```python
from build123d import *

# Parameters (mm, degrees)
SKETCH1_W                = 220
SKETCH1_H                = 170
BOSS_EXTRUDE1_DEPTH      = 100
SKETCH3_W                = 200
SKETCH3_H                = 150
CUT_EXTRUDE2_DEPTH       = 90
FILLET1_R                = 10
SKETCH4_W                = 130
SKETCH4_H                = 90
CUT_EXTRUDE3_DEPTH       = 10
SKETCH8_W                = 223.528125383
SKETCH8_H                = 171.877504909
CUT_EXTRUDE5_DEPTH       = 10
CUT_EXTRUDE7_REACH       = 505.38
SKETCH9_R                = 7.5
CUT_EXTRUDE8_REACH       = 505.38
SKETCH10_W               = 50
SKETCH10_H               = 30
CUT_EXTRUDE9_REACH       = 384.733
SKETCH11_W               = 20
SKETCH11_H               = 1
CUT_EXTRUDE10_REACH      = 505.38
CUT_EXTRUDE11_DEPTH      = 10
CUT_EXTRUDE12_REACH      = 505.38
SKETCH15_R               = 5.863278905
CUT_EXTRUDE13_DEPTH      = 8
BOSS_EXTRUDE3_DEPTH      = 8
BOSS_EXTRUDE3_DEPTH_BACK = 3
SKETCH16_R               = 1.3
SKETCH17_R               = 13.825952239
SKETCH17_R_2             = 5.825952239
EXTRUDE_THIN1_DEPTH      = 8
FILLET2_R                = 8
SKETCH18_W               = 15
SKETCH18_H               = 21
CUT_EXTRUDE14_DEPTH      = 249


with BuildPart() as part:
    # Sketch1 → Boss-Extrude1 (new body)
    with BuildSketch(Plane.XY):
        with Locations((-355.179344655, 214.973620006)):
            Rectangle(SKETCH1_W, SKETCH1_H)
    extrude(amount=BOSS_EXTRUDE1_DEPTH)

    # Sketch3 → Cut-Extrude2 (cut)
    with BuildSketch(Plane.XY.offset(100)):
        with Locations((-355.179344655, 214.973620006)):
            Rectangle(SKETCH3_W, SKETCH3_H)
    extrude(amount=-CUT_EXTRUDE2_DEPTH, mode=Mode.SUBTRACT)

    # Fillet1
    fillet1_edges = [part.edges().sort_by_distance(p)[0] for p in [
        (-355.179344655, 299.973620006, 0),
        (-245.179344655, 214.973620006, 0),
        (-355.179344655, 129.973620006, 0),
        (-465.179344655, 214.973620006, 0),
    ]]
    fillet(fillet1_edges, radius=FILLET1_R)

    # Sketch4 → Cut-Extrude3 (cut)
    with BuildSketch(Plane(origin=(0, 299.973620006, 0), x_dir=(1, 0, 0), z_dir=(0, 1, 0))):
        with Locations((-330.179344655, -55)):
            Rectangle(SKETCH4_W, SKETCH4_H)
    extrude(amount=-CUT_EXTRUDE3_DEPTH, mode=Mode.SUBTRACT)

    # Sketch8 → Cut-Extrude5 (cut)
    with BuildSketch(Plane.XY.offset(90)):
        with Locations((-354.80209528, 215.143634814)):
            Rectangle(SKETCH8_W, SKETCH8_H)
    extrude(amount=CUT_EXTRUDE5_DEPTH, mode=Mode.SUBTRACT)

    # Sketch9 → Cut-Extrude7 (cut, up to next)
    with BuildSketch(Plane.XZ.offset(-129.973620006), mode=Mode.PRIVATE) as cut_extrude7_sk1:
        with Locations(Location((-445.179344655, 30, 0), (0, 0, 270))):
            Circle(SKETCH9_R)
    cut_extrude7_tool1 = extrude(cut_extrude7_sk1.sketch, amount=-CUT_EXTRUDE7_REACH, mode=Mode.PRIVATE) & part.part
    add(cut_extrude7_tool1.solids().sort_by_distance((-445.179345, 129.97362, 30))[0], mode=Mode.SUBTRACT)

    # Sketch10 → Cut-Extrude8 (cut, up to next)
    with BuildSketch(Plane.XZ.offset(-129.973620006), mode=Mode.PRIVATE) as cut_extrude8_sk1:
        with Locations((-282.179344655, 35)):
            Rectangle(SKETCH10_W, SKETCH10_H)
    cut_extrude8_tool1 = extrude(cut_extrude8_sk1.sketch, amount=-CUT_EXTRUDE8_REACH, mode=Mode.PRIVATE) & part.part
    add(cut_extrude8_tool1.solids().sort_by_distance((-282.179345, 129.97362, 35))[0], mode=Mode.SUBTRACT)

    # Sketch11 → Cut-Extrude9 (cut, up to next)
    with BuildSketch(Plane.ZY.offset(465.179344655), mode=Mode.PRIVATE) as cut_extrude9_sk1:
        with Locations((30.04058668, 161.535899553)):
            Rectangle(SKETCH11_W, SKETCH11_H)
    cut_extrude9_tool1 = extrude(cut_extrude9_sk1.sketch, amount=-CUT_EXTRUDE9_REACH, mode=Mode.PRIVATE) & part.part
    # Sketch11 → Cut-Extrude9 (cut, up to next)
    with BuildSketch(Plane.ZY.offset(465.179344655), mode=Mode.PRIVATE) as cut_extrude9_sk2:
        with Locations((30.04058668, 156.535899553)):
            Rectangle(SKETCH11_W, SKETCH11_H)
    cut_extrude9_tool2 = extrude(cut_extrude9_sk2.sketch, amount=-CUT_EXTRUDE9_REACH, mode=Mode.PRIVATE) & part.part
    # Sketch11 → Cut-Extrude9 (cut, up to next)
    with BuildSketch(Plane.ZY.offset(465.179344655), mode=Mode.PRIVATE) as cut_extrude9_sk3:
        with Locations((30.04058668, 166.535899553)):
            Rectangle(SKETCH11_W, SKETCH11_H)
    cut_extrude9_tool3 = extrude(cut_extrude9_sk3.sketch, amount=-CUT_EXTRUDE9_REACH, mode=Mode.PRIVATE) & part.part
    # Sketch11 → Cut-Extrude9 (cut, up to next)
    with BuildSketch(Plane.ZY.offset(465.179344655), mode=Mode.PRIVATE) as cut_extrude9_sk4:
        with Locations((30.04058668, 171.535899553)):
            Rectangle(SKETCH11_W, SKETCH11_H)
    cut_extrude9_tool4 = extrude(cut_extrude9_sk4.sketch, amount=-CUT_EXTRUDE9_REACH, mode=Mode.PRIVATE) & part.part
    # Sketch11 → Cut-Extrude9 (cut, up to next)
    with BuildSketch(Plane.ZY.offset(465.179344655), mode=Mode.PRIVATE) as cut_extrude9_sk5:
        with Locations((30.04058668, 176.535899553)):
            Rectangle(SKETCH11_W, SKETCH11_H)
    cut_extrude9_tool5 = extrude(cut_extrude9_sk5.sketch, amount=-CUT_EXTRUDE9_REACH, mode=Mode.PRIVATE) & part.part
    add(cut_extrude9_tool1.solids().sort_by_distance((-465.179345, 161.5359, 30.040587))[0], mode=Mode.SUBTRACT)
    add(cut_extrude9_tool2.solids().sort_by_distance((-465.179345, 156.5359, 30.040587))[0], mode=Mode.SUBTRACT)
    add(cut_extrude9_tool3.solids().sort_by_distance((-465.179345, 166.5359, 30.040587))[0], mode=Mode.SUBTRACT)
    add(cut_extrude9_tool4.solids().sort_by_distance((-465.179345, 171.5359, 30.040587))[0], mode=Mode.SUBTRACT)
    add(cut_extrude9_tool5.solids().sort_by_distance((-465.179345, 176.5359, 30.040587))[0], mode=Mode.SUBTRACT)

    # Sketch12 → Cut-Extrude10 (cut, up to next)
    with BuildSketch(Plane.XZ.offset(-129.973620006), mode=Mode.PRIVATE) as cut_extrude10_sk1:
        Polygon((-354.097719845, 36.683084204), (-334.097719845, 36.683084204), (-327.697719845, 29.055861211), (-335.358164277, 22.627985114), (-352.790666107, 22.627985114), (-360.497719845, 29.023338287), align=None)
    cut_extrude10_tool1 = extrude(cut_extrude10_sk1.sketch, amount=-CUT_EXTRUDE10_REACH, mode=Mode.PRIVATE) & part.part
    add(cut_extrude10_tool1.solids().sort_by_distance((-344.093749, 129.97362, 29.715571))[0], mode=Mode.SUBTRACT)

    # Sketch13 → Cut-Extrude11 (cut)
    with BuildSketch(Plane.XZ.offset(-129.973620006)):
        Polygon((-360.497719845, 29.023338287), (-354.110242897, 21.329175679), (-354.11397805, 22.529175679), (-354.117713203, 23.729175679), align=None)
        Polygon((-334.045816465, 21.329175679), (-327.697719845, 29.055861211), (-334.045816465, 23.729175679), (-334.045816465, 22.627985114), align=None)
    extrude(amount=-CUT_EXTRUDE11_DEPTH, mode=Mode.SUBTRACT)

    # Sketch14 → Cut-Extrude12 (cut, up to next)
    with BuildSketch(Plane.XZ.offset(-129.973620006), mode=Mode.PRIVATE) as cut_extrude12_sk1:
        Polygon((-354.117713203, 23.729175679), (-354.110242897, 21.329175679), (-334.045816465, 21.329175679), (-334.045816465, 23.729175679), align=None)
    cut_extrude12_tool1 = extrude(cut_extrude12_sk1.sketch, amount=-CUT_EXTRUDE12_REACH, mode=Mode.PRIVATE) & part.part
    add(cut_extrude12_tool1.solids().sort_by_distance((-344.079897, 129.97362, 22.52925))[0], mode=Mode.SUBTRACT)

    # Sketch15 → Cut-Extrude13 (cut)
    with BuildSketch(Plane.XZ.offset(-129.973620006)):
        with Locations(Location((-385.408718364, 29.414099171, 0), (0, 0, 270))):
            Circle(SKETCH15_R)
    extrude(amount=-CUT_EXTRUDE13_DEPTH, mode=Mode.SUBTRACT)

    # Sketch16 → Boss-Extrude3 (add, two sides: drawn at the far end of the back side and taken through both)
    with BuildSketch(Plane.XZ.offset(-137.973620006).offset(-BOSS_EXTRUDE3_DEPTH_BACK)):
        with Locations(Location((-385.408718364, 29.414099171, 0), (0, 0, 270))):
            Circle(SKETCH16_R)
    extrude(amount=BOSS_EXTRUDE3_DEPTH + BOSS_EXTRUDE3_DEPTH_BACK)

    # Sketch17 → Extrude-Thin1 (add)
    with BuildSketch(Plane.XZ.offset(-129.973620006)):
        with Locations((-385.408718364, 29.414099171)):
            Circle(SKETCH17_R)
        with Locations((-385.408718364, 29.414099171)):
            Circle(SKETCH17_R_2, mode=Mode.SUBTRACT)
    extrude(amount=EXTRUDE_THIN1_DEPTH)

    # Fillet2
    fillet2_edges = [part.edges().sort_by_distance(p)[0] for p in [
        (-399.234670603, 121.973620006, 29.414099171),
    ]]
    fillet(fillet2_edges, radius=FILLET2_R - 0.0001)  # a hair under: the kernel refuses the full size

    # Sketch18 → Cut-Extrude14 (cut)
    with BuildSketch(Plane(origin=(-245.179344655, 0, 0), x_dir=(0, 0, -1), z_dir=(1, 0, 0))):
        with Locations((-24.5, 200.473620006)):
            Rectangle(SKETCH18_W, SKETCH18_H)
    extrude(amount=-CUT_EXTRUDE14_DEPTH, mode=Mode.SUBTRACT)


solid = part.part
```
Geometry: final body of the model. Coordinates: model frame, mm. A direction names the side the tool comes from. Round coordinates to 2 decimals unless told otherwise and drop trailing zeros. Write each loop counter-clockwise with the first axis right and the second up, starting at its lowest first coordinate (ties: lowest second). Pieces come first, ordered by that corner, then holes.
Item 1: Pin query (flat end, axial travel): P1, Ø11, axis at x = -462, z = 30, coming from the -Y side; P2, Ø12, axis at x = -377.5, z = 71, coming from the +Y side; P3, Ø5, axis at x = -261, z = 36.5, coming from the -Y side. Return the tip coordinate at first contact, or that it passes through.
Item 2: Section query B-B (y = 206). Return loops of the section in (x, z), plus the area to 3 significant figures.
Item 3: Section query A-A (x = -350). Return loops of the section in (y, z), plus the area to 3 significant figures.
Item 4: Section query D-D (z = 68.5). Return loops of the section in (x, y).
Item 5: Set-up query: faces 4 (the face through (-307.179, 135, 35)), 5 (the face through (-460, 162.036, 30)), 6 (the face through (-460, 189.974, 25)), 7 (the face through (-260, 289.974, 51)). Return all of +Z, -Z, +X, -X, +Y, -Y with unobstructed straight access to the full face (end or side cutting, diameter ignored); none if empty.
Item 6: Mould query, pull axis Y, two halves, no side actions, for faces 1 (the face through (-353.639, 297.122, 3.007)), 2 (the face through (-452.5, 134.9, 31.63)), 3 (the face through (-460, 200, 32)). Classes: +Y half, -Y half, draft (parallel to the pull), parting line (faces both ways), or undercut.
Item 7: Material intervals for L1, parallel to X at y = 243, z = 58; L2, parallel to Y at x = -406.5, z = 29; L3, parallel to Z at x = -451.5, y = 230.5, sorted ascending.
Item 8: Section query C-C (y = 247.5). Return loops of the section in (x, z).
Completed:
1. P1: stops at y = 129.97
1. P2: stops at y = 139.97
1. P3: stops at y = 289.97
2. outline: (-465.18, 10) arc R10 ccw to (-455.18, 0) - (-255.18, 0) arc R10 ccw to (-245.18, 10) - (-245.18, 17) - (-255.18, 17) - (-255.18, 10) - (-455.18, 10) - (-455.18, 17) - (-465.18, 17) - close; (-465.18, 32) - (-455.18, 32) - (-455.18, 90) - (-465.18, 90) - close; (-255.18, 32) - (-245.18, 32) - (-245.18, 90) - (-255.18, 90) - close
2. area: 3,460 mm2
3. outline: (129.97, 10) arc R10 ccw to (139.97, 0) - (289.97, 0) arc R10 ccw to (299.97, 10) - (139.97, 10) - (139.97, 21.33) - (129.97, 21.33) - close; (129.97, 36.68) - (139.97, 36.68) - (139.97, 90) - (129.97, 90) - close
3. area: 2,300 mm2
4. outline: (-465.18, 129.97) - (-245.18, 129.97) - (-245.18, 299.97) - (-265.18, 299.97) - (-265.18, 289.97) - (-255.18, 289.97) - (-255.18, 139.97) - (-455.18, 139.97) - (-455.18, 289.97) - (-395.18, 289.97) - (-395.18, 299.97) - (-465.18, 299.97) - close
5. face 4: +Y, -Y
5. face 5: -X
5. face 6: +X, -X
5. face 7: +Z
6. face 1: +Y half
6. face 2: draft
6. face 3: undercut
7. L1: x = -465.18 to -455.18, -255.18 to -245.18
7. L2: y = 129.97 to 139.97, 289.97 to 299.97
7. L3: z = 0 to 10
8. outline: (-465.18, 10) arc R10 ccw to (-455.18, 0) - (-255.18, 0) arc R10 ccw to (-245.18, 10) - (-245.18, 90) - (-255.18, 90) - (-255.18, 10) - (-455.18, 10) - (-455.18, 90) - (-465.18, 90) - close
